Here's the drawing with two shaded views (mm, measured from the low corner). I have some questions. A direction names the side the tool comes from. Give positions to 0.01 mm unless a question says otherwise; leave off trailing zeros. Write each loop counter-clockwise with the first axis right and the second up, starting at its lowest first coordinate (ties: lowest second). Pieces come first, ordered by that corner, then holes.
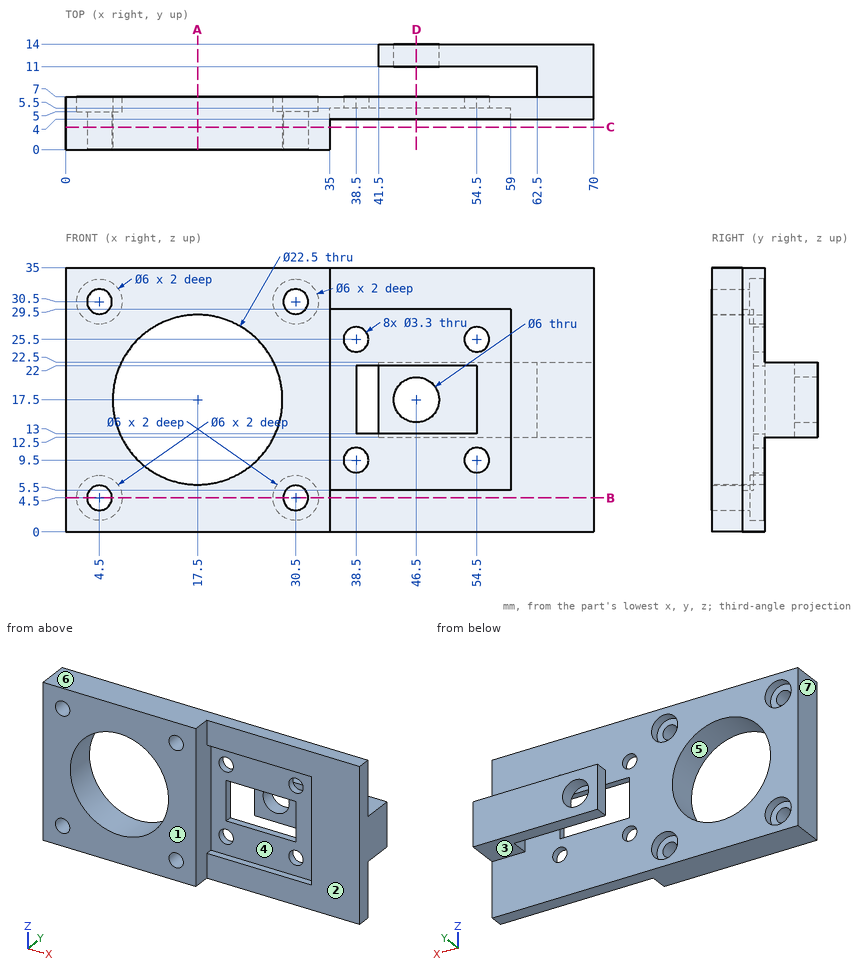
1) Suppose I cut it at A-A on x = 17.5. Write out the boundary of the cut face in (y, z), plus the area to 3 significant figures.
Values follow:
outline: (0, 0) - (7, 0) - (7, 6.25) - (0, 6.25) - close; (0, 28.75) - (7, 28.75) - (7, 35) - (0, 35) - close
area: 87.5 mm2
2) Suppose I cut it at D-D on x = 46.5. Write out the boundary of the cut face in (y, z).
Values follow:
outline: (4, 0) - (7, 0) - (7, 13) - (5.5, 13) - (5.5, 5.5) - (4, 5.5) - close; (4, 29.5) - (5.5, 29.5) - (5.5, 22) - (7, 22) - (7, 35) - (4, 35) - close; (11, 12.5) - (14, 12.5) - (14, 14.5) - (11, 14.5) - close; (11, 20.5) - (14, 20.5) - (14, 22.5) - (11, 22.5) - close
3) If we mould it in two halves opening along X, with no side actions, what happens to the marked faces 4, 5, 6 and 7? For each: +X half, -X half, draft (parallel to the pull), parting line (faces both ways), or undercut.
Values follow:
face 4: undercut
face 5: undercut
face 6: draft
face 7: -X half
4) Suppose I cut it at B-B on z = 4.5. Write out the boundary of the cut face in (x, y).
Values follow:
outline: (0, 0) - (2.85, 0) - (2.85, 5) - (1.5, 5) - (1.5, 7) - (0, 7) - close; (6.15, 0) - (28.85, 0) - (28.85, 5) - (27.5, 5) - (27.5, 7) - (7.5, 7) - (7.5, 5) - (6.15, 5) - close; (32.15, 0) - (35, 0) - (35, 4) - (70, 4) - (70, 7) - (33.5, 7) - (33.5, 5) - (32.15, 5) - close
5) For the marked faces 1, 2 and 3, which set-ups out of +Z, -Z, +X, -X, +Y, -Y let a thin tool reach every point of the face, with its end or its side?
Values follow:
face 1: +Z, -Z, +X, -X, -Y
face 2: +Z, -Z, +X, -Y
face 3: -Z, +X, -X, +Y
6) Please list where these lines run through material, in increasing order: L1, parallel to X at y = 5.55, z = 4.5; L2, parallel to X at y = 5, z = 17; L3, parallel to X at y = 12.25, z = 17.5.
Values follow:
L1: x = 0 to 1.5, 7.5 to 27.5, 33.5 to 70
L2: x = 0 to 6.26, 28.74 to 35, 59 to 70
L3: x = 41.5 to 43.5, 49.5 to 70
7) Suppose I cut it at C-C on y = 3. Write out the boundary of the cut face in (x, z), plus the area to 3 significant figures.
Values follow:
outline: (0, 0) - (35, 0) - (35, 35) - (0, 35) - close; hole circle Ø3.3 at (4.5, 4.5); hole circle Ø3.3 at (4.5, 30.5); hole circle Ø22.5 at (17.5, 17.5); hole circle Ø3.3 at (30.5, 4.5); hole circle Ø3.3 at (30.5, 30.5)
area: 793 mm2
8) For pin 1 Ø2.5 at (x, z) = (30.5, 30.5) entering from -Y; pin 2 Ø1.8 at (x, z) = (30.5, 5.5) entering from +Y; pin 3 Ø3 at (x, y) = (41, 10) entering from -Z; pin 4 Ø5 at (x, z) = (5.5, 30.5) entering from +Y, each with a flat end and sliding along its axis, tell me the tip position at first contact or that it passes through.
Values follow:
pin 1: passes through
pin 2: stops at y = 5
pin 3: stops at z = 12.5
pin 4: stops at y = 7
